```python
from build123d import *

# Parameters (mm, degrees)
SKETCH1_R                = 32
BOSS_EXTRUDE1_DEPTH      = 0.999998
SKETCH2_R                = 32
SKETCH2_R_2              = 30.05
BOSS_EXTRUDE2_DEPTH      = 4
M4_CLEARANCE_HOLE1_D     = 4.8
M4_CLEARANCE_HOLE1_DEPTH = 1.999996


with BuildPart() as part:
    # Sketch1 → Boss-Extrude1 (new body, symmetric)
    with BuildSketch(Plane.XY):
        Circle(SKETCH1_R)
    extrude(amount=BOSS_EXTRUDE1_DEPTH, both=True)

    # Sketch2 → Boss-Extrude2 (add)
    with BuildSketch(Plane.XY.offset(0.999998)):
        Circle(SKETCH2_R)
        Circle(SKETCH2_R_2, mode=Mode.SUBTRACT)
    extrude(amount=BOSS_EXTRUDE2_DEPTH)

    # M4 Clearance Hole1
    with Locations(Plane(origin=(0, 0, -0.999998), x_dir=(-1, 0, 0), z_dir=(0, 0, -1))):
        with Locations((0, 17.4498), (0, -17.4498)):
            Hole(M4_CLEARANCE_HOLE1_D / 2, depth=M4_CLEARANCE_HOLE1_DEPTH)


solid = part.part
```
Read the model definition and answer for the solid it produces. Units are mm, in the model's axes. A direction names the side the tool comes from. Give positions to 0.01 mm unless a question says otherwise; leave off trailing zeros. Write each loop counter-clockwise with the first axis right and the second up, starting at its lowest first coordinate (ties: lowest second). Pieces come first, ordered by that corner, then holes. Notation, with made-up numbers: (52.25, 59) - (74.25, 59) arc R24 ccw to (74.25, 92) - close; hole circle Ø9 at (48.25, 64.25). An arc over 180 degrees is marked (long way). Write item = value, one per line. Start each with the question number.
Item 1: Find section D-D (x = 15). Give the vertices of the cut face in (y, z).
Item 2: A tool of negligible diameter and unlimited length cuts with its end or side. For faces 1 (the flat face through (0, 0, -1)), 2 (the flat face through (0, 0, 1)), from which of +Z, -Z, +X, -X, +Y, -Y can it reach the whole face along a straight path? Write none if from no direction.
Item 3: Each of these flat-tipped pins is pushed along its axis until it touches: P1, Ø2, axis at x = 23.5, z = 0.5, coming from the -Y side; P2, Ø6, axis at x = -15, y = 18, coming from the +Z side; P3, Ø4.5, axis at x = 0, y = -17.45, coming from the +Z side. Where does it stop, or does it pass through?
Item 4: Find section B-B (y = 0). Give the vertices of the cut face in (x, z), then the cut area to 3 significant figures.
Item 5: The mould has two halves that part along Y. Classify faces 3 (the cylindrical face through (-30.02, 1.32, 2.97)), 4 (the flat face through (-29, -9, 5)), 5 (the cylindrical face through (-6.94, -31.24, 1.96)): +Y half, -Y half, draft (parallel to the pull), parting line (faces both ways), or undercut.
Item 6: Find section C-C (z = 3.1). Give the vertices of the cut face in (x, y).
Item 7: Find the intervals of material crossed by probe 1 along Y at (x, z) = (0, -0.5); probe 2 along X at (y, z) = (1, 2.25); probe 3 along Y at (x, z) = (0, 1.8), in increasing order. Write a range as [from, to].
Item 8: Find section A-A (x = 0). Give the vertices of the cut face in (y, z), then the cut area to 3 significant figures.
Response:
q1.outline = (-28.27, -1) - (28.27, -1) - (28.27, 5) - (26.04, 5) - (26.04, 1) - (-26.04, 1) - (-26.04, 5) - (-28.27, 5) - close
q2.face_1 = -Z, +X, -X, +Y, -Y
q2.face_2 = +Z
q3.P1 = -22.75
q3.P2 = 1
q3.P3 = through
q4.outline = (-32, -1) - (32, -1) - (32, 5) - (30.05, 5) - (30.05, 1) - (-30.05, 1) - (-30.05, 5) - (-32, 5) - close
q4.area = 144 mm²
q5.face_3 = undercut
q5.face_4 = draft
q5.face_5 = parting line
q6.outline = circle Ø64 at (0, 0); hole circle Ø60.1 at (0, 0)
q7.probe_1 = [-32, -19.85], [-15.05, 15.05], [19.85, 32]
q7.probe_2 = [-31.98, -30.03], [30.03, 31.98]
q7.probe_3 = [-32, -30.05], [30.05, 32]
q8.outline = (-32, -1) - (-19.85, -1) - (-19.85, 1) - (-30.05, 1) - (-30.05, 5) - (-32, 5) - close; (-15.05, -1) - (15.05, -1) - (15.05, 1) - (-15.05, 1) - close; (19.85, -1) - (32, -1) - (32, 5) - (30.05, 5) - (30.05, 1) - (19.85, 1) - close
q8.area = 124 mm²
